```python
from build123d import *

# Parameters (mm, degrees)
SKETCH1_W          = 6.35
SKETCH1_H          = 1.4224
CHAMFER1_SIZE      = 0.47625
SKETCH4_R          = 2.7051
EXTRUDE1_DEPTH     = 1.4986
CUT_EXTRUDE1_DEPTH = 0.7493
SKETCH7_R          = 0.916543552
CUT_EXTRUDE4_DEPTH = 0.7493
CUT_EXTRUDE4_TAPER = 45
SKETCH8_R          = 0.79375
CUT_EXTRUDE5_DEPTH = 0.249766667
CUT_EXTRUDE5_TAPER = 60


with BuildPart() as part:
    # Sketch1 → Revolve1 (revolve)
    with BuildSketch(Plane(origin=(0, 0, 0), x_dir=(0, 0, -1), z_dir=(1, 0, 0))):
        with Locations((3.175, 0.7112)):
            Rectangle(SKETCH1_W, SKETCH1_H)
    revolve(axis=Axis((0, 0, 0), (0, 0, 1)))

    # Chamfer1
    chamfer1_edges = [part.edges().sort_by_distance(p)[0] for p in [
        (0, -1.4224, -6.35),
    ]]
    chamfer(chamfer1_edges, length=CHAMFER1_SIZE)

    # Sketch4 → Extrude1 (add)
    with BuildSketch(Plane.XY):
        Circle(SKETCH4_R)
    extrude(amount=EXTRUDE1_DEPTH)

    # Sketch9 → Cut-Revolve3 (revolve, cut)
    with BuildSketch(Plane(origin=(0, 0, 0), x_dir=(0, 0, -1), z_dir=(1, 0, 0))):
        with BuildLine():
            Line((0, 2.7051), (-0.381, 2.7051))
            ThreePointArc((-0.381, 2.7051), (-1.025093234, 2.138064897), (-1.4986, 1.4224))
            Line((-1.4986, 1.4224), (-1.8796, 1.4224))
            Line((-1.8796, 1.4224), (-1.8796, 3.0861))
            Line((-1.8796, 3.0861), (0, 3.0861))
            Line((0, 3.0861), (0, 2.7051))
        make_face()
    revolve(axis=Axis((0, 0, 0), (0, 0, 1)), mode=Mode.SUBTRACT)

    # Sketch6 → Cut-Extrude1 (cut)
    with BuildSketch(Plane.XY.offset(1.4986)):
        Polygon((0, -0.916543552), (0.79375, -0.458271776), (0.79375, 0.458271776), (0, 0.916543552), (-0.79375, 0.458271776), (-0.79375, -0.458271776), align=None)
    extrude(amount=-CUT_EXTRUDE1_DEPTH, mode=Mode.SUBTRACT)

    # Sketch7 → Cut-Extrude4 (cut)
    with BuildSketch(Plane.XY.offset(1.4986)):
        Circle(SKETCH7_R)
    extrude(amount=-CUT_EXTRUDE4_DEPTH, taper=CUT_EXTRUDE4_TAPER, mode=Mode.SUBTRACT)

    # Sketch8 → Cut-Extrude5 (cut)
    with BuildSketch(Plane.XY.offset(0.7493)):
        Circle(SKETCH8_R)
    extrude(amount=-CUT_EXTRUDE5_DEPTH, taper=CUT_EXTRUDE5_TAPER, mode=Mode.SUBTRACT)


solid = part.part
```
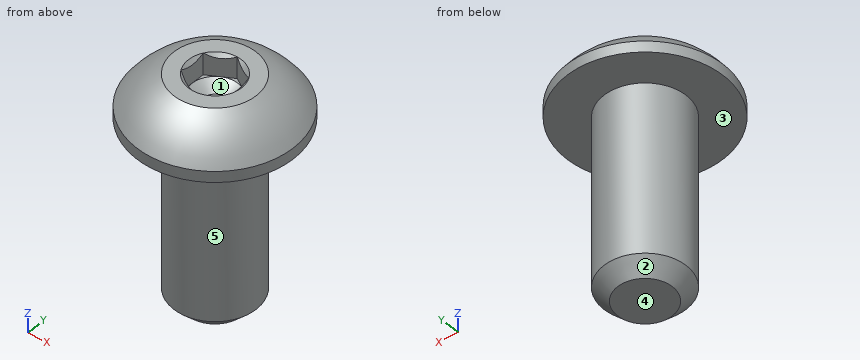
Build history of the part. All positions in model axes, mm. Face numbers are marked on the shaded views. A direction names the side the tool comes from. Give positions to 0.01 mm unless a question says otherwise; leave off trailing zeros. Order: outer loops, then holes, each group sorted by start corner. A loop starts at its lowest first (then second) coordinate and runs counter-clockwise, first axis right, second up. Notation, with made-up numbers: M 8,8 L 13,8 A20 ccw 13,16 Z; hole C 40,-27.75 d3. An arc over 180 degrees is marked long. Return JSON: item names as keys, results as strings.
Q1. Band-saw the part on B-B (x = -2.2). Give the cut face in (y, z).
Answer list:
{"outline": "M -1.57,0 L 1.57,0 L 1.57,0.38 A2.4 ccw -1.57,0.38 Z"}
Q2. 3-axis set-ups, long thin cutter, end or side, ignore diameter. For the marked faces 4 and 5: which of +Z, -Z, +X, -X, +Y, -Y reach the whole face in a straight line?
Answer list:
{"face 4": "-Z, +X, -X, +Y, -Y", "face 5": "-Z"}
Q3. Band-saw the part on C-C (y = 1.75). Give the cut face in (x, z), then the cut area to 3 significant figures.
Answer list:
{"outline": "M -2.06,0 L 2.06,0 L 2.06,0.38 A2.74 ccw -2.06,0.38 Z", "area": "4.24 mm^2"}
Q4. Flat gauge pins, fed straight in: pin 1 (1.5 mm diameter, centred on x = -1, y = -2, fed in from +Z); pin 2 (0.8 mm diameter, centred on y = 0, z = 1.5, fed in from +X); pin 3 (1.5 mm diameter, centred on y = 1, z = -1.5, fed in from +X). Where does each tip first touch, or does it go through?
Answer list:
{"pin 1": "stops at z = 1.47", "pin 2": "stops at x = 2.05", "pin 3": "stops at x = 1.4"}
Q5. Two-plate mould, pull along X, no slides. Class the marked faces 1, 2 and 3: pulls with the +X half, pulls with the -X half, needs draft (parallel to the pull), parting line crosses it, or undercut.
Answer list:
{"face 1": "undercut", "face 2": "parting line crosses it", "face 3": "needs draft"}
Q6. Band-saw the part on A-A (z = -4.5). Give the cut face in (x, y).
Answer list:
{"outline": "C 0,0 d2.84"}
Q7. Wall check: probe 1 along X at (y, z) = (0.05, -1.5); probe 2 along Z at (x, y) = (0.05, 1.55); probe 3 along Y at (x, z) = (-0.35, -3.75). Give the ranges that are in metal, low to high. Write a range as from..to.
Answer list:
{"probe 1": "x = -1.42..1.42", "probe 2": "z = 0..1.43", "probe 3": "y = -1.38..1.38"}
